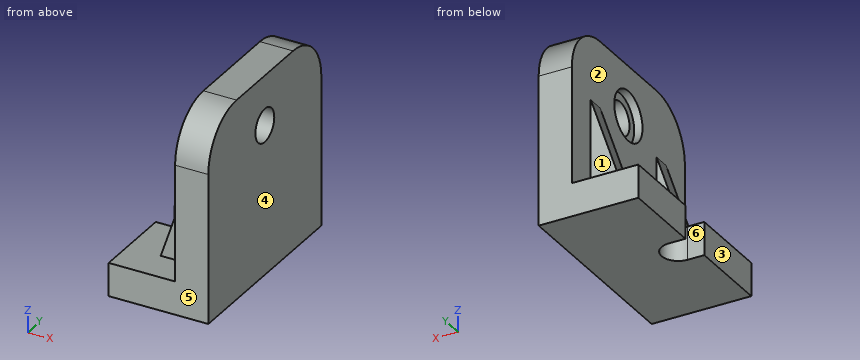
```python
from build123d import *

# Parameters (mm, degrees)
F1_DEPTH  = 76.2
F2_R      = 12.7
F3_DEPTH  = 76.201
F5_DEPTH  = 25.401
F6_R      = 38.1
F7_R      = 19.05
F7_R_2    = 12.7
F8_DEPTH  = 6.35
F11_DEPTH = 6.35


# Not quite as in the source:
# - a pattern or mirror of a feature is missing from the dataset's text; its kind, count and spacing are read off the source's solid


with BuildPart() as f1:
    # F0 (on Front) → F1 (new body, symmetric)
    with BuildSketch(Plane.XZ):
        Polygon((-76.2, 0), (0, 0), (0, 152.4), (-25.4, 152.4), (-25.4, 25.4), (-76.2, 25.4), align=None)
    extrude(amount=F1_DEPTH, both=True)

    # F2 (on face) → F3 (cut, through all)
    with BuildSketch(Plane.YZ):
        with Locations((0, 114.3)):
            Circle(F2_R)
    extrude(amount=-F3_DEPTH, mode=Mode.SUBTRACT)

    # F4 (on face) → F5 (cut, through all)
    with BuildSketch(Plane.XY.offset(25.4)):
        with BuildLine():
            Line((-63.5, 12.7), (-76.2, 12.7))
            Line((-76.2, 12.7), (-76.2, -12.7))
            Line((-76.2, -12.7), (-63.5, -12.7))
            ThreePointArc((-63.5, -12.7), (-50.8, 0), (-63.5, 12.7))
        make_face()
    extrude(amount=-F5_DEPTH, mode=Mode.SUBTRACT)

    # F6
    f6_edges = [f1.edges().sort_by_distance(p)[0] for p in [
        (-12.7, -76.2, 152.4),
        (-12.7, 76.2, 152.4),
    ]]
    fillet(f6_edges, radius=F6_R)

    # F7 (on face) → F8 (cut)
    with BuildSketch(Plane(origin=(-25.4, 0, 0), x_dir=(0, -1, 0), z_dir=(-1, 0, 0))):
        with Locations((0, 114.3)):
            Circle(F7_R)
        with Locations((0, 114.3)):
            Circle(F7_R_2, mode=Mode.SUBTRACT)
    extrude(amount=-F8_DEPTH, mode=Mode.SUBTRACT)

    # F10 (on offset) → F11 (join, symmetric)
    with BuildSketch(Plane.XZ.offset(44.45)):
        Polygon((-50.8, 25.4), (-25.4, 25.4), (-25.4, 101.6), align=None)
    f11 = extrude(amount=F11_DEPTH, both=True)

    # F11_copies: F11 across plane
    add(f11.mirror(Plane.ZX))


solid = f1.part
```
Input: part model. Units: mm. Frame: model coordinates. Face numbers are marked on the shaded views. A direction names the side the tool comes from. Coordinates: 2 decimals unless noted, no trailing zeros. Loops run counter-clockwise (first coordinate to the right, second up) from the corner with the lowest first, then second, coordinate; pieces in that order, holes last. Notation, with made-up numbers: (-29.75, 56) - (11.25, 56) arc R23 cw to (11.25, 75) - close; hole circle Ø4 at (-40, -20). An arc over 180 degrees is marked (long way). Answer in a Markdown table with one row per item.
(1) Material intervals for L1, parallel to Z at x = -10, y = 0; L2, parallel to Y at x = -32, z = 73.5; L3, parallel to Y at x = -20, z = 114, sorted ascending. Write a range as from..to.
Model answer:
| item | result |
|---|---|
| L1 | z = 0..101.6, 127..152.4 |
| L2 | y = -50.8..-38.1, 38.1..50.8 |
| L3 | y = -76.2..-19.05, 19.05..76.2 |
(2) Pin query (flat end, axial travel): P1, Ø12.5, axis at x = -42.5, z = 65, coming from the -Y side; P2, Ø1, axis at y = 18, z = 72.5, coming from the -X side; P3, Ø23, axis at y = 0, z = 114.3, coming from the +X side. Return the tip coordinate at first contact, or that it passes through.
Model answer:
| item | result |
|---|---|
| P1 | stops at y = -50.8 |
| P2 | stops at x = -25.4 |
| P3 | passes through |
(3) Set-up query: the marked faces 1, 2 and 3. Return all of +Z, -Z, +X, -X, +Y, -Y with unobstructed straight access to the full face (end or side cutting, diameter ignored); none if empty.
Model answer:
| item | result |
|---|---|
| face 1 | +Z, -X, +Y |
| face 2 | +Z, -X |
| face 3 | +Z, -Z, -X, +Y, -Y |
(4) Cut plane B-B on z = 56. Output: boundary loops of the cut face in (x, y).
Model answer:
| item | result |
|---|---|
| outline | (-40.6, -50.8) - (-25.4, -50.8) - (-25.4, -76.2) - (0, -76.2) - (0, 76.2) - (-25.4, 76.2) - (-25.4, 50.8) - (-40.6, 50.8) - (-40.6, 38.1) - (-25.4, 38.1) - (-25.4, -38.1) - (-40.6, -38.1) - close |
(5) Mould query, pull axis Y, two halves, no side actions, for the marked faces 4, 5 and 6. Classes: pulls with the +Y half, pulls with the -Y half, needs draft (parallel to the pull), parting line crosses it, or undercut.
Model answer:
| item | result |
|---|---|
| face 4 | needs draft |
| face 5 | pulls with the -Y half |
| face 6 | undercut |
(6) Cut plane A-A on y = 0. Output: boundary loops of the cut face in (x, z).
Model answer:
| item | result |
|---|---|
| outline | (-50.8, 0) - (0, 0) - (0, 101.6) - (-19.05, 101.6) - (-19.05, 95.25) - (-25.4, 95.25) - (-25.4, 25.4) - (-50.8, 25.4) - close; (-25.4, 133.35) - (-19.05, 133.35) - (-19.05, 127) - (0, 127) - (0, 152.4) - (-25.4, 152.4) - close |
(7) Cut plane D-D on y = -34. Output: boundary loops of the cut face in (x, z).
Model answer:
| item | result |
|---|---|
| outline | (-76.2, 0) - (0, 0) - (0, 152.4) - (-25.4, 152.4) - (-25.4, 25.4) - (-76.2, 25.4) - close |
(8) Cut plane C-C on x = -33. Output: boundary loops of the cut face in (y, z), plus the area to 3 significant figures.
Model answer:
| item | result |
|---|---|
| outline | (-76.2, 0) - (76.2, 0) - (76.2, 25.4) - (50.8, 25.4) - (50.8, 78.8) - (38.1, 78.8) - (38.1, 25.4) - (-38.1, 25.4) - (-38.1, 78.8) - (-50.8, 78.8) - (-50.8, 25.4) - (-76.2, 25.4) - close |
| area | 5,230 mm² |
